Here's how the part is built. I have some questions about the finished solid (model axes, mm). A direction names the side the tool comes from. Coordinates: 2 decimals unless noted, no trailing zeros. Write each loop counter-clockwise with the first axis right and the second up, starting at its lowest first coordinate (ties: lowest second). Pieces come first, ordered by that corner, then holes. Notation, with made-up numbers: (-4, -25.5) -> (13, -25.5) arc R29 cw to (13, 1.5) -> close; hole circle Ø8 at (79.25, 70.5). An arc over 180 degrees is marked (long way). Put each result on its own line as item: value.
```python
from build123d import *

# Parameters (mm, degrees)
BOSS_EXTRUDE1_DEPTH      = 10
BOSS_EXTRUDE1_DEPTH_BACK = 100
SKETCH2_W                = 100
SKETCH2_H                = 100
SKETCH3_R                = 20.704608813
BOSS_EXTRUDE2_DEPTH      = 100
SKETCH4_W                = 61.706837877
SKETCH4_H                = 40.386202863
CUT_EXTRUDE1_DEPTH       = 207.155281281


with BuildPart() as part:
    # Sketch2 → Boss-Extrude1 (new, two sides: drawn at the far end of the back side and taken through both)
    with BuildSketch(Plane.XY.offset(-BOSS_EXTRUDE1_DEPTH_BACK)):
        Rectangle(SKETCH2_W, SKETCH2_H)
    extrude(amount=BOSS_EXTRUDE1_DEPTH + BOSS_EXTRUDE1_DEPTH_BACK)

    # Sketch3 → Boss-Extrude2 (add)
    with BuildSketch(Plane(origin=(50, 0, 0), x_dir=(0, 0, -1), z_dir=(1, 0, 0))):
        with Locations(Location((45.530604039, 0, 0), (0, 0, 180))):
            Circle(SKETCH3_R)
    extrude(amount=BOSS_EXTRUDE2_DEPTH)

    # Sketch4 → Cut-Extrude1 (cut, through all)
    with BuildSketch(Plane(origin=(0, 50, 0), x_dir=(1, 0, 0), z_dir=(0, 1, 0))):
        with Locations((-1.559035635, 44.897496948)):
            Rectangle(SKETCH4_W, SKETCH4_H)
    extrude(amount=-CUT_EXTRUDE1_DEPTH, mode=Mode.SUBTRACT)


solid = part.part
```
Item 1: Imagine slicing it at D-D on y = -38.5. Write out the boundary of the cut face in (x, z), then the cut area to 3 significant figures.
Output:
outline: (-50, -100) -> (50, -100) -> (50, 10) -> (-50, 10) -> close; hole (-32.41, -65.09) -> (29.29, -65.09) -> (29.29, -24.7) -> (-32.41, -24.7) -> close
area: 8,510 mm²
Item 2: Which directions (+Z, -Z, +X, -X, +Y, -Y) give clear straight access to the entire face, cutting with the end or side of a thin tool? Please do faces 4 (the flat face through (50, -23, -46)), 5 (the flat face through (-2, 1, -65.091)), 6 (the flat face through (-1, -50, -70)).
Output:
face 4: +X
face 5: +Y, -Y
face 6: +Z, -Z, +X, -X, -Y
Item 3: For P1, Ø8, axis at x = 98, y = -15.5, coming from the +Z side; P2, Ø3, axis at x = 68, z = -54.5, coming from the -Y side; P3, Ø4, axis at y = 13, z = -62.5, coming from the +X side; P4, Ø1.5, axis at x = 51, z = -36.5, coming from the -Y side, each with a flat end and sliding along its axis, tell me the tip position at first contact or that it passes through.
Output:
P1: stops at z = -28.31
P2: stops at y = -19.31
P3: stops at x = 150
P4: stops at y = -18.98
Item 4: Please list where these lines run through material, in increasing order: line 1 along X through (y, z) = (27.5, -58); line 2 along Z through (x, y) = (24, 18); line 3 along X through (y, z) = (-17, -6). Write a range as from..to.
Output:
line 1: x = -50..-32.41, 29.29..50
line 2: z = -100..-65.09, -24.7..10
line 3: x = -50..50
Item 5: If we mould it in two halves opening along Z, with no side actions, what happens to faces 1 (the flat face through (-2, 1, -24.704)), 2 (the flat face through (-1, 1, 10)), 3 (the flat face through (150, 0, -46))? For each: released by +Z, released by -Z, zero draft, split by the parting line, or undercut.
Output:
face 1: undercut
face 2: released by +Z
face 3: zero draft
Item 6: Imagine slicing it at B-B on y = 0. Write out the boundary of the cut face in (x, z), then the cut area to 3 significant figures.
Output:
outline: (-50, -100) -> (50, -100) -> (50, -66.24) -> (150, -66.24) -> (150, -24.83) -> (50, -24.83) -> (50, 10) -> (-50, 10) -> close; hole (-32.41, -65.09) -> (29.29, -65.09) -> (29.29, -24.7) -> (-32.41, -24.7) -> close
area: 12,600 mm²
Item 7: Imagine slicing it at C-C on z = -35. Write out the boundary of the cut face in (x, y), then the cut area to 3 significant figures.
Output:
outline: (-50, -50) -> (-32.41, -50) -> (-32.41, 50) -> (-50, 50) -> close; (29.29, -50) -> (50, -50) -> (50, -17.83) -> (150, -17.83) -> (150, 17.83) -> (50, 17.83) -> (50, 50) -> (29.29, 50) -> close
area: 7,390 mm²
Item 8: Imagine slicing it at A-A on x = 0.5. Write out the boundary of the cut face in (y, z).
Output:
outline: (-50, -100) -> (50, -100) -> (50, -65.09) -> (-50, -65.09) -> close; (-50, -24.7) -> (50, -24.7) -> (50, 10) -> (-50, 10) -> close
